Work out the finished part from the listing and answer in its coordinate system (mm). Face numbers are marked on the shaded views. A direction names the side the tool comes from. Round coordinates to 2 decimals unless told otherwise and drop trailing zeros. Write each loop counter-clockwise with the first axis right and the second up, starting at its lowest first coordinate (ties: lowest second). Pieces come first, ordered by that corner, then holes. Notation, with made-up numbers: M 29,8.25 L 83,8.25 A21 cw 83,46.25 Z; hole C 3.5,-15.5 d10. An arc over 180 degrees is marked long. Answer in a Markdown table with one row per item.
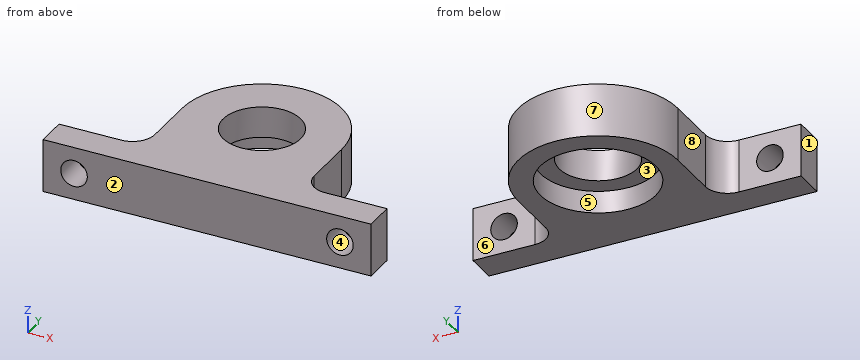
```python
from build123d import *

# Parameters (mm, degrees)
SKETCH1_R           = 8.75
BOSS_EXTRUDE1_DEPTH = 12
SKETCH2_R           = 3
CUT_EXTRUDE1_DEPTH  = 8
SKETCH3_R           = 13
CUT_EXTRUDE2_DEPTH  = 5
BOSS_EXTRUDE2_DEPTH = 12
FILLET2_R           = 5


with BuildPart() as part:
    # Sketch1 → Boss-Extrude1 (new body)
    with BuildSketch(Plane.XY):
        with BuildLine():
            Line((-5.916079783, -17), (-37, -17))
            Line((-37, -17), (-37, -24))
            Line((-37, -24), (0, -24))
            Line((0, -24), (37, -24))
            Line((37, -24), (37, -17))
            Line((37, -17), (5.916079783, -17))
            ThreePointArc((5.916079783, -17), (0, 18), (-5.916079783, -17))
        make_face()
        Circle(SKETCH1_R, mode=Mode.SUBTRACT)
    extrude(amount=BOSS_EXTRUDE1_DEPTH)

    # Sketch2 → Cut-Extrude1 (cut, through all)
    with BuildSketch(Plane(origin=(0, -17, 0), x_dir=(1, 0, 0), z_dir=(0, 1, 0))):
        with Locations((30, -6)):
            Circle(SKETCH2_R)
        with Locations((-30, -6)):
            Circle(SKETCH2_R)
    extrude(amount=-CUT_EXTRUDE1_DEPTH, mode=Mode.SUBTRACT)

    # Sketch3 → Cut-Extrude2 (cut)
    with BuildSketch(Plane(origin=(0, 0, 0), x_dir=(-1, 0, 0), z_dir=(0, 0, -1))):
        Circle(SKETCH3_R)
    extrude(amount=-CUT_EXTRUDE2_DEPTH, mode=Mode.SUBTRACT)

    # Sketch4 → Boss-Extrude2 (add, through all)
    with BuildSketch(Plane(origin=(0, 0, 0), x_dir=(-1, 0, 0), z_dir=(0, 0, -1))):
        Polygon((-18, 0), (-5.916079783, -17), (-18, -17), align=None)
        Polygon((18, 0), (18, -17), (5.916079783, -17), align=None)
    extrude(amount=-BOSS_EXTRUDE2_DEPTH)

    # Fillet2
    fillet2_edges = [part.edges().sort_by_distance(p)[0] for p in [
        (-18, -17, 6),
        (18, -17, 6),
    ]]
    fillet(fillet2_edges, radius=FILLET2_R)


solid = part.part
```
1. Determine the mould class of the marked faces 1, 2, 3 and 4 for opening direction X: released by +X, released by -X, zero draft, split by the parting line, or undercut.
Calculated:
| item | result |
|---|---|
| face 1 | released by -X |
| face 2 | zero draft |
| face 3 | undercut |
| face 4 | undercut |
2. The part is cut by section A-A (x = 30). Determine the outline of the cut face in (y, z), plus the area to 3 significant figures.
Calculated:
| item | result |
|---|---|
| outline | M -24,0 L -17,0 L -17,3 L -24,3 Z; M -24,9 L -17,9 L -17,12 L -24,12 Z |
| area | 42.0 mm² |
3. Consider line 1 along X through (y, z) = (-20.5, 6); line 2 along Z through (x, y) = (30, -18); line 3 along Y through (x, z) = (0, 10.5). Determine where each line is inside the solid, lowest interval first. Write a range as from..to.
Calculated:
| item | result |
|---|---|
| line 1 | x = -37..-33, -27..27, 33..37 |
| line 2 | z = 0..3, 9..12 |
| line 3 | y = -24..-8.75, 8.75..18 |
4. The part is cut by section C-C (y = -18). Determine the outline of the cut face in (x, z), plus the area to 3 significant figures.
Calculated:
| item | result |
|---|---|
| outline | M -37,0 L 37,0 L 37,12 L -37,12 Z; hole C -30,6 d6; hole C 30,6 d6 |
| area | 831 mm² |
5. The part is cut by section D-D (x = 0). Determine the outline of the cut face in (y, z).
Calculated:
| item | result |
|---|---|
| outline | M -24,0 L -13,0 L -13,5 L -8.75,5 L -8.75,12 L -24,12 Z; M 8.75,5 L 13,5 L 13,0 L 18,0 L 18,12 L 8.75,12 Z |
6. Given pin 1 (6 mm diameter, centred on x = -18, z = 9, fed in from +Y); pin 2 (1 mm diameter, centred on x = -19.5, z = 9, fed in from +Y); pin 3 (2 mm diameter, centred on x = 5.5, z = 7.5, fed in from +Y), each flat-ended and moving along its own axis, determine where each tip first touches the part or whether it passes through.
Calculated:
| item | result |
|---|---|
| pin 1 | stops at y = 9.95 |
| pin 2 | stops at y = -15 |
| pin 3 | stops at y = 17.43 |
7. A tool of negligible diameter and unlimited length cuts with its end or side. For the marked faces 5, 6, 7 and 8, from which of +Z, -Z, +X, -X, +Y, -Y can it reach the whole face along a straight path? Write none if from no direction.
Calculated:
| item | result |
|---|---|
| face 5 | -Z |
| face 6 | +Z, -Z, +X, +Y |
| face 7 | +Z, -Z, +Y |
| face 8 | +Z, -Z, -X, +Y |
8. The part is cut by section B-B (z = 9.75). Determine the outline of the cut face in (x, y).
Calculated:
| item | result |
|---|---|
| outline | M -37,-24 L 37,-24 L 37,-17 L 23,-17 A5 cw 18,-12 L 18,0 A18 ccw -18,0 L -18,-12 A5 cw -23,-17 L -37,-17 Z; hole C 0,0 d17.5 |
